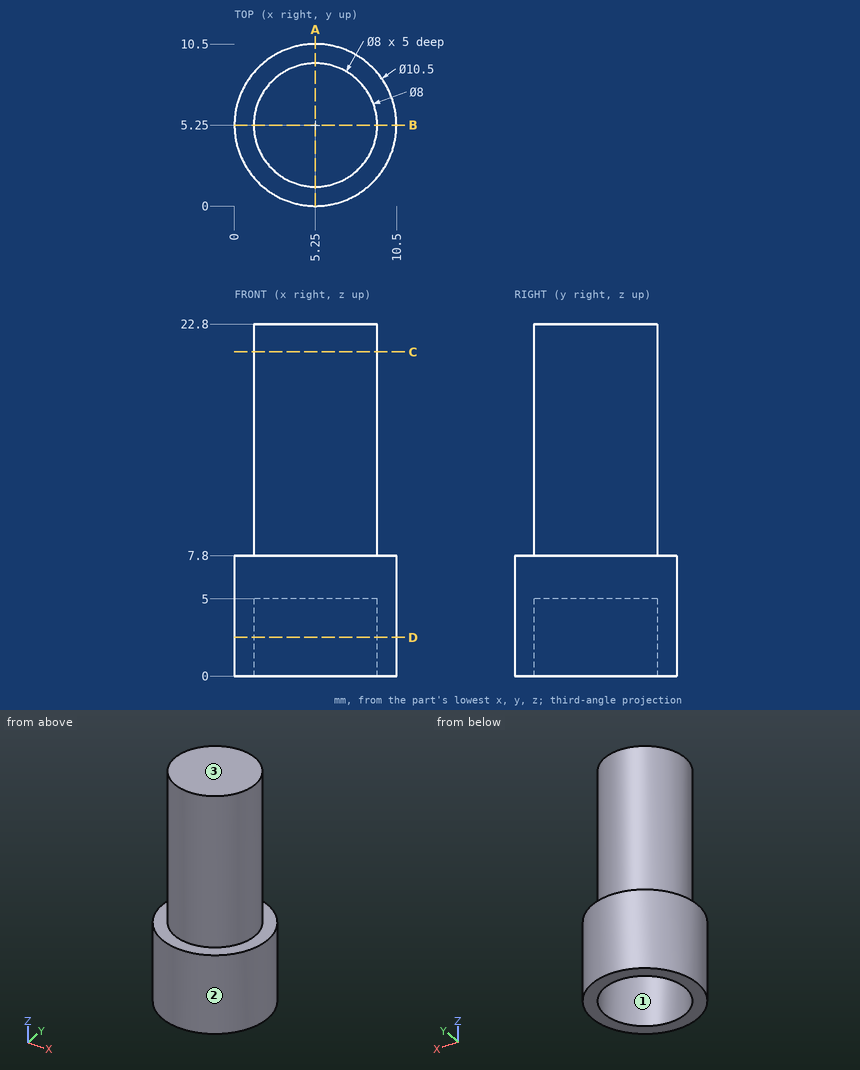
Design review of the part shown in the three views and the two pictorial views. Dimensions are in mm from the part's minimum x, y and z. Round coordinates to 2 decimals unless told otherwise and drop trailing zeros. Loops run counter-clockwise (first coordinate to the right, second up) from the corner with the lowest first, then second, coordinate; pieces in that order, holes last. Notation, with made-up numbers: M -14.75,57.25 L 32.25,57.25 A15 cw 32.25,77.25 Z; hole C 65,26 d6. An arc over 180 degrees is marked long. Put each result on its own line as item: value.
Q1. Consider section C-C, the plane z = 21. Give the boundary of the cut face in (x, y).
Result set:
outline: C 5.25,5.25 d8
Q2. Consider section D-D, the plane z = 2.5. Give the boundary of the cut face in (x, y), then the cut area to 3 significant figures.
Result set:
outline: C 5.25,5.25 d10.5; hole C 5.25,5.25 d8
area: 36.3 mm²
Q3. Mouldability with a two-part tool opening along Y and no side actions: class the marked faces 1, 2 and 3 as released by +Y, released by -Y, zero draft, split by the parting line, or undercut.
Result set:
face 1: undercut
face 2: split by the parting line
face 3: zero draft
Q4. To check wall thickness, follow L1, parallel to Y at x = 5.25, z = 3.3; L2, parallel to Z at x = 6.5, y = 3.5; L3, parallel to X at y = 6.5, z = 4.25. State the ranges of each line that lie inside material, in increasing order.
Result set:
L1: y = 0 to 1.25, 9.25 to 10.5
L2: z = 5 to 22.8
L3: x = 0.15 to 1.45, 9.05 to 10.35
Q5. For pin 1 (4 mm diameter, centred on y = 3, z = 6, fed in from -X); pin 2 (1.5 mm diameter, centred on y = 7.5, z = 3.5, fed in from +X); pin 3 (1 mm diameter, centred on x = 1.5, z = 9.5, fed in from +Y), all flat-tipped, find the tip position at first contact; note any pin that passes through.
Result set:
pin 1: stops at x = 0.01
pin 2: stops at x = 10.28
pin 3: stops at y = 7.58
Q6. Consider section A-A, the plane x = 5.25. Give the boundary of the cut face in (y, z), then the cut area to 3 significant figures.
Result set:
outline: M 0,0 L 1.25,0 L 1.25,5 L 9.25,5 L 9.25,0 L 10.5,0 L 10.5,7.8 L 9.25,7.8 L 9.25,22.8 L 1.25,22.8 L 1.25,7.8 L 0,7.8 Z
area: 162 mm²
